Verification items for the finished model (mm, model axes). A direction names the side the tool comes from. Coordinates: 2 decimals unless noted, no trailing zeros. Write each loop counter-clockwise with the first axis right and the second up, starting at its lowest first coordinate (ties: lowest second). Pieces come first, ordered by that corner, then holes. Notation, with made-up numbers: M -19.5,73.5 L 13.5,73.5 A26 cw 13.5,111.5 Z; hole C 53,-5 d2. An arc over 180 degrees is marked long. One line per item, written item: value.
```python
from build123d import *

# Parameters (mm, degrees)
F0_W      = 26
F0_H      = 20
F1_DEPTH  = 4
F2_W      = 26
F2_H      = 6
F3_DEPTH  = 5
F4_R      = 1.9
F5_DEPTH  = 25
F6_W      = 11.2
F6_H      = 6
F7_DEPTH  = 5
F8_R      = 2.6
F9_DEPTH  = 4
F10_R     = 2.6
F11_DEPTH = 3
F12_R     = 1


# Not quite as in the source:
# - a fillet or chamfer that OpenCascade refuses, or shapes differently, is made with other operations: its cross-section is extruded or revolved along the edge and cut away or added
# - a feature names something its author has since deleted; it is built from what else it names


with BuildPart() as f1:
    # F0 (on Top) → F1 (new body)
    with BuildSketch(Plane.XY):
        with Locations((13, 0)):
            Rectangle(F0_W, F0_H)
    extrude(amount=F1_DEPTH)

    # F2 (on face) → F3 (join)
    with BuildSketch(Plane.XY.offset(4)):
        with Locations((13, 0)):
            Rectangle(F2_W, F2_H)
    extrude(amount=F3_DEPTH)

    # F4 (on face) → F5 (cut)
    with BuildSketch(Plane.XY.offset(9)):
        with Locations((5, 0)):
            Circle(F4_R)
    extrude(amount=-F5_DEPTH, mode=Mode.SUBTRACT)

    # F6 (on face) → F7 (cut, through all)
    with BuildSketch(Plane.XY.offset(9)):
        with Locations((20.5, 0)):
            Rectangle(F6_W, F6_H)
    extrude(amount=-F7_DEPTH, mode=Mode.SUBTRACT)

    # F8 (on face) → F9 (cut, through all)
    with BuildSketch(Plane.XY.offset(4)):
        with Locations((20.5, 0)):
            Circle(F8_R)
    extrude(amount=-F9_DEPTH, mode=Mode.SUBTRACT)

    # F10 (on face) → F11 (join)
    with BuildSketch(Plane(origin=(0, 0, 0), x_dir=(0, -1, 0), z_dir=(-1, 0, 0))):
        Polygon((-10, 24), (-10, 4), (-3, 4), (-3, 9), (3, 9), (3, 4), (10, 4), (10, 24), align=None)
        with Locations((0, 14)):
            Circle(F10_R, mode=Mode.SUBTRACT)
        Polygon((-10, 4), (-10, 0), (10, 0), (10, 4), (3, 4), (3, 9), (-3, 9), (-3, 4), align=None)
    extrude(amount=F11_DEPTH)

    # F12
    f12_edges = [f1.edges().sort_by_distance(p)[0] for p in [
        (-1.5, -10, 24),
        (-1.5, 10, 24),
        (11.5, -10, 0),
        (11.5, 10, 0),
    ]]
    fillet(f12_edges, radius=F12_R)

    # F13: chamfer of 0.5 x 0.2886751346 on 1 edges, made by hand

    # F13_s1 → F13_t2 (revolve, cut)
    with BuildSketch(Plane.XZ):
        Polygon((7.1886751346, 0), (6.9, 0.5), (6.9, 0), align=None)
    revolve(axis=Axis((5, 0, 0), (0, 0, 1)), mode=Mode.SUBTRACT)


solid = f1.part
```
Item 1: Cross-section at A-A, the plane z = 4.75. Enter the section's corners in (x, y).
The answers:
outline: M -3,-10 L 0,-10 L 0,-3 L 14.9,-3 L 14.9,3 L 0,3 L 0,10 L -3,10 Z; hole C 5,0 d3.8
Item 2: Access from +Z, -Z, +X, -X, +Y, -Y to the whole of each face (thin tool, end or side, straight path). Record for faces 5 (the face through (7, 3, 6)), 6 (the face through (22.98, 0.78, 2.03)), 7 (the face through (7, -3, 6)), 8 (the face through (7.3, 0, 9)), 9 (the face through (11.297, -9.715, 0.301)).
The answers:
face 5: +Z, +X, +Y
face 6: +Z, -Z
face 7: +Z, +X, -Y
face 8: +Z, +X, +Y, -Y
face 9: -Z, +X, -X, -Y
Item 3: Cross-section at D-D, the plane y = 0. Enter the section's corners in (x, z).
The answers:
outline: M -3,0 L 2.81,0 L 3.1,0.5 L 3.1,9 L 0,9 L 0,11.4 L -3,11.4 Z; M -3,16.6 L 0,16.6 L 0,24 L -3,24 Z; M 6.9,0.5 L 7.19,0 L 17.9,0 L 17.9,4 L 14.9,4 L 14.9,9 L 6.9,9 Z; M 23.1,0 L 26,0 L 26,4 L 23.1,4 Z
Item 4: Cross-section at C-C, the plane z = 14. Enter the section's corners in (x, y), and give its area (3 significant figures).
The answers:
outline: M -3,-10 L 0,-10 L 0,-2.6 L -3,-2.6 Z; M -3,2.6 L 0,2.6 L 0,10 L -3,10 Z
area: 44.4 mm²
Item 5: Cross-section at B-B, the plane x = 20.5. Enter the section's corners in (y, z), and give its area (3 significant figures).
The answers:
outline: M -10,1 A1 ccw -9,0 L -2.6,0 L -2.6,4 L -10,4 Z; M 2.6,0 L 9,0 A1 ccw 10,1 L 10,4 L 2.6,4 Z
area: 58.8 mm²
Item 6: Scan lines: line 1 (Z direction, x = -1.65, y = 0); line 2 (Y direction, x = 5, z = 2.5); line 3 (Y direction, x = 20.5, z = 1.9). Record each from-to range of solid material in increasing order.
The answers:
line 1: z = 0 to 11.4, 16.6 to 24
line 2: y = -10 to -1.9, 1.9 to 10
line 3: y = -10 to -2.6, 2.6 to 10
Item 7: Draft check along Y on faces 1 (the face through (3.1, 0.08, 4.81)), 2 (the face through (-1.48, 0.56, 11.46)), 3 (the face through (16, 0, 4)), 4 (the face through (7.3, -10, 3.8)). Enter one of: released by +Y, released by -Y, zero draft, split by the parting line, or undercut.
The answers:
face 1: undercut
face 2: undercut
face 3: zero draft
face 4: released by -Y
Item 8: Go/stop test with flat-tipped pins: P1, Ø1.5, axis at x = 15.5, y = -6, coming from the +Z side; P2, Ø1.5, axis at y = -1, z = 7, coming from the +X side; P3, Ø8, axis at x = 5, z = 10, coming from the -Y side. Record where each tip stops, or that it passes through.
The answers:
P1: stops at z = 4
P2: stops at x = 14.9
P3: stops at y = -3
